from build123d import *

# Parameters (mm, degrees)
SKETCH1_W                                       = 78
SKETCH1_H                                       = 69
BOSS_EXTRUDE1_DEPTH                             = 11
SKETCH4_W                                       = 18
SKETCH4_H                                       = 45
CUT_EXTRUDE2_DEPTH                              = 6.5
SKETCH5_W                                       = 7.8
SKETCH5_H                                       = 2.7
CUT_EXTRUDE3_DEPTH                              = 4.5
SKETCH6_W                                       = 26
SKETCH6_H                                       = 64
CUT_EXTRUDE4_DEPTH                              = 4
SKETCH8_R                                       = 1.5
CUT_EXTRUDE5_DEPTH                              = 73.645065829
CSK_FOR_12_FLAT_HEAD_MACHINE_SCREW1_D           = 5.7912
CSK_FOR_12_FLAT_HEAD_MACHINE_SCREW1_CSINK_D     = 11.1252
CSK_FOR_12_FLAT_HEAD_MACHINE_SCREW1_CSINK_ANGLE = 82
SKETCH24_W                                      = 35.5
SKETCH24_H                                      = 19.8
CUT_EXTRUDE7_DEPTH                              = 74.138947144


with BuildPart() as part:
    # Sketch1 → Boss-Extrude1 (new body)
    with BuildSketch(Plane(origin=(0, 0, 0), x_dir=(1, 0, 0), z_dir=(0, 1, 0))):
        with Locations((-15.96214511, -12.483701367)):
            Rectangle(SKETCH1_W, SKETCH1_H)
    extrude(amount=BOSS_EXTRUDE1_DEPTH)

    # Sketch4 → Cut-Extrude2 (cut)
    with BuildSketch(Plane(origin=(0, 11, 0), x_dir=(1, 0, 0), z_dir=(0, 1, 0))):
        with Locations((-27.96214511, -21.783701367)):
            Rectangle(SKETCH4_W, SKETCH4_H)
    extrude(amount=-CUT_EXTRUDE2_DEPTH, mode=Mode.SUBTRACT)

    # Sketch5 → Cut-Extrude3 (cut)
    with BuildSketch(Plane(origin=(0, 11, 0), x_dir=(1, 0, 0), z_dir=(0, 1, 0))):
        with Locations((-27.96214511, -45.633701367)):
            Rectangle(SKETCH5_W, SKETCH5_H)
    extrude(amount=-CUT_EXTRUDE3_DEPTH, mode=Mode.SUBTRACT)

    # Sketch6 → Cut-Extrude4 (cut)
    with BuildSketch(Plane(origin=(0, 11, 0), x_dir=(1, 0, 0), z_dir=(0, 1, 0))):
        with Locations((-4.96214511, -11.983701367)):
            Rectangle(SKETCH6_W, SKETCH6_H)
    extrude(amount=-CUT_EXTRUDE4_DEPTH, mode=Mode.SUBTRACT)

    # Sketch8 → Cut-Extrude5 (cut, through all)
    with BuildSketch(Plane(origin=(0, 7, 0), x_dir=(1, 0, 0), z_dir=(0, 1, 0))):
        with Locations(Location((5.03785489, -40.483701367, 0), (0, 0, 270))):
            Circle(SKETCH8_R)
        with Locations(Location((-14.96214511, -40.483701367, 0), (0, 0, 270))):
            Circle(SKETCH8_R)
        with Locations(Location((-14.96214511, 15.516298633, 0), (0, 0, 270))):
            Circle(SKETCH8_R)
        with Locations(Location((5.03785489, 15.516298633, 0), (0, 0, 270))):
            Circle(SKETCH8_R)
    extrude(amount=-CUT_EXTRUDE5_DEPTH, mode=Mode.SUBTRACT)

    # CSK for #12 Flat Head Machine Screw1 (through all)
    with Locations(Plane(origin=(0, 11, 0), x_dir=(1, 0, 0), z_dir=(0, 1, 0))):
        with Locations((-49.46214511, -38.983701367), (-49.46214511, -9.983701367), (17.53785489, -9.983701367)):
            CounterSinkHole(CSK_FOR_12_FLAT_HEAD_MACHINE_SCREW1_D / 2, CSK_FOR_12_FLAT_HEAD_MACHINE_SCREW1_CSINK_D / 2, counter_sink_angle=CSK_FOR_12_FLAT_HEAD_MACHINE_SCREW1_CSINK_ANGLE)

    # Sketch24 → Cut-Extrude7 (cut, through all)
    with BuildSketch(Plane(origin=(0, 11, 0), x_dir=(1, 0, 0), z_dir=(0, 1, 0))):
        with Locations((-37.21214511, 12.116298633)):
            Rectangle(SKETCH24_W, SKETCH24_H)
    extrude(amount=-CUT_EXTRUDE7_DEPTH, mode=Mode.SUBTRACT)


solid = part.part
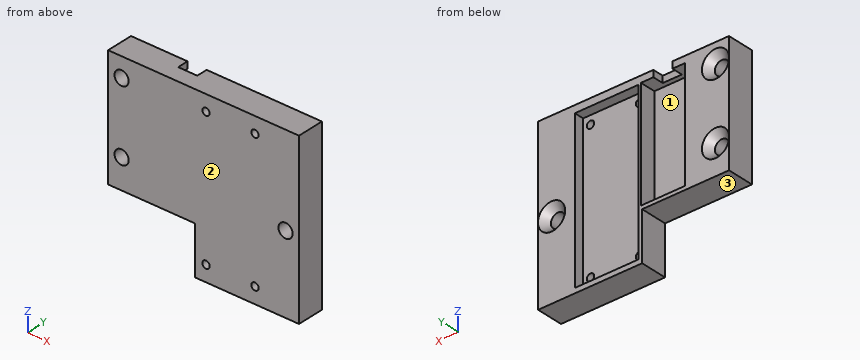
Could you check a few things on this model? Use its own coordinates, in mm. Face numbers are marked on the shaded views. A direction names the side the tool comes from. Give positions to 0.01 mm unless a question says otherwise; leave off trailing zeros. Order: outer loops, then holes, each group sorted by start corner. A loop starts at its lowest first (then second) coordinate and runs counter-clockwise, first axis right, second up. Notation, with made-up numbers: (73, -26) -> (89, -26) arc R20 ccw to (89, 1) -> close; hole circle Ø1 at (43.5, 38). An arc over 180 degrees is marked (long way). Answer in a Markdown table with one row per item. Add a question column.
Item 1: Imagine slicing it at B-B (z = -3.5). List the corners of the cut face in (x, y) for me, and give its area (4 significant figures).
Item 2: Please list where these lines run through material, in increasing order: probe 1 along X at (y, z) = (9, 19); probe 2 along X at (y, z) = (6.75, 36); probe 3 along X at (y, z) = (8.25, -16.5).
Item 3: For the marked faces 1, 2 and 3, which set-ups out of +Z, -Z, +X, -X, +Y, -Y let a thin tool reach every point of the face, with its end or its side?
Item 4: Imagine slicing it at A-A (x = -6). List the corners of the cut face in (y, z) for me, and give its area (3 significant figures).
Item 5: Imagine slicing it at C-C (y = 2.25). List the corners of the cut face in (x, z) for me, and give its area (3 significant figures).
Item 6: I'm going to push flat-ended pins straight in: P1, Ø1.4, axis at x = -27, z = 45.5, coming from the +Y side; P2, Ø5, axis at x = -26, y = 6.5, coming from the -Z side; P3, Ø9, axis at x = -30.5, z = 25, coming from the +Y side. Where does each tip first touch, or does it pass through?
Item 7: Imagine slicing it at D-D (y = 9.5). List the corners of the cut face in (x, z) for me, and give its area (3 significant figures).
Result:
| question | item | result |
|---|---|---|
| 1 | outline | (-19.46, 0) -> (23.04, 0) -> (23.04, 11) -> (8.04, 11) -> (8.04, 7) -> (-17.96, 7) -> (-17.96, 11) -> (-19.46, 11) -> close |
| 1 | area | 363.5 mm2 |
| 2 | probe 1 | -54.96 to -36.96, -18.96 to -17.96, 8.04 to 23.04 |
| 2 | probe 2 | -54.96 to -36.96, -18.96 to 23.04 |
| 2 | probe 3 | -19.46 to -17.96, 8.04 to 23.04 |
| 3 | face 1 | +Y |
| 3 | face 2 | +Z, -Z, +X, -X, -Y |
| 3 | face 3 | -Z, -X, +Y, -Y |
| 4 | outline | (0, -22.02) -> (11, -22.02) -> (11, -20.02) -> (7, -20.02) -> (7, 43.98) -> (11, 43.98) -> (11, 46.98) -> (0, 46.98) -> close |
| 4 | area | 503 mm2 |
| 5 | outline | (-54.96, -2.22) -> (-19.46, -2.22) -> (-19.46, -22.02) -> (23.04, -22.02) -> (23.04, 46.98) -> (-54.96, 46.98) -> close; hole circle Ø5.79 at (-49.46, 9.98); hole circle Ø5.79 at (-49.46, 38.98); hole circle Ø3 at (-14.96, -15.52); hole circle Ø3 at (-14.96, 40.48); hole circle Ø3 at (5.04, -15.52); hole circle Ø3 at (5.04, 40.48); hole circle Ø5.79 at (17.54, 9.98) |
| 5 | area | 4,570 mm2 |
| 6 | P1 | y = 6.5 |
| 6 | P2 | z = -2.22 |
| 6 | P3 | y = 4.5 |
| 7 | outline | (-54.96, -2.22) -> (-19.46, -2.22) -> (-19.46, -22.02) -> (23.04, -22.02) -> (23.04, 46.98) -> (-24.06, 46.98) -> (-24.06, 44.28) -> (-18.96, 44.28) -> (-18.96, -0.72) -> (-36.96, -0.72) -> (-36.96, 44.28) -> (-31.86, 44.28) -> (-31.86, 46.98) -> (-54.96, 46.98) -> close; hole circle Ø8.52 at (-49.46, 9.98); hole circle Ø8.52 at (-49.46, 38.98); hole (-17.96, -20.02) -> (8.04, -20.02) -> (8.04, 43.98) -> (-17.96, 43.98) -> close; hole circle Ø8.52 at (17.54, 9.98) |
| 7 | area | 2,010 mm2 |
